Input: part model. Units: mm. Frame: model coordinates. Face numbers are marked on the shaded views. A direction names the side the tool comes from. Coordinates: 2 decimals unless noted, no trailing zeros. Loops run counter-clockwise (first coordinate to the right, second up) from the corner with the lowest first, then second, coordinate; pieces in that order, holes last. Notation, with made-up numbers: (40, -20) -> (55, -20) arc R25 cw to (55, 14) -> close; hole circle Ø5 at (37, 26). An arc over 180 degrees is marked (long way). Put each result on its own line as item: value. Start each with the question number.
1) Set-up query: the marked faces 1 and 2. Return all of +Z, -Z, +X, -X, +Y, -Y with unobstructed straight access to the full face (end or side cutting, diameter ignored); none if empty.
2) Contact query for flat-ended pins moving along their axis: P1, Ø3, axis at y = -1.5, z = 3, coming from the +X side; P2, Ø1, axis at y = -0.5, z = 2.5, coming from the -X side. Output: stop coordinate, or through.
3) Cut plane C-C (z = 4.75). Return the cut outline in (x, y), plus the area to 3 significant figures.
4) Material intervals for L1, parallel to Z at x = -1.65, y = -0.6; L2, parallel to Y at x = 0, z = 4.5; L3, parallel to Y at x = 0.85, z = 4.75, sorted ascending.
5) Cut plane A-A (x = 0). Return the cut outline in (y, z).
from build123d import *

# Parameters (mm, degrees)
SKETCH1_R           = 1.5
BOSS_EXTRUDE1_DEPTH = 6.5
CHAMFER1_SIZE       = 0.1
SKETCH2_R           = 2.5
BOSS_EXTRUDE2_DEPTH = 1
CHAMFER2_SIZE       = 0.2


with BuildPart() as part:
    # Sketch1 → Boss-Extrude1 (new body)
    with BuildSketch(Plane.XY):
        Circle(SKETCH1_R)
    extrude(amount=BOSS_EXTRUDE1_DEPTH)

    # Chamfer1
    chamfer1_edges = [part.edges().sort_by_distance(p)[0] for p in [
        (-1.5, 0, 0),
    ]]
    chamfer(chamfer1_edges, length=CHAMFER1_SIZE)

    # Sketch2 → Boss-Extrude2 (add)
    with BuildSketch(Plane.XY.offset(6.5)):
        Circle(SKETCH2_R)
    extrude(amount=BOSS_EXTRUDE2_DEPTH)

    # Chamfer2
    chamfer2_edges = [part.edges().sort_by_distance(p)[0] for p in [
        (-2.5, 0, 7.5),
    ]]
    chamfer(chamfer2_edges, length=CHAMFER2_SIZE)


solid = part.part
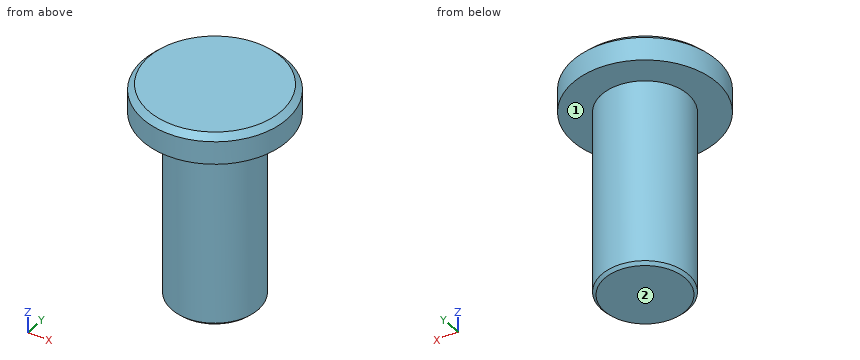
Results found:
1. face 1: -Z
1. face 2: -Z, +X, -X, +Y, -Y
2. P1: stops at x = 1.5
2. P2: stops at x = -1.5
3. outline: circle Ø3 at (0, 0)
3. area: 7.07 mm2
4. L1: z = 6.5 to 7.5
4. L2: y = -1.5 to 1.5
4. L3: y = -1.24 to 1.24
5. outline: (-2.5, 6.5) -> (-1.5, 6.5) -> (-1.5, 0.1) -> (-1.4, 0) -> (1.4, 0) -> (1.5, 0.1) -> (1.5, 6.5) -> (2.5, 6.5) -> (2.5, 7.3) -> (2.3, 7.5) -> (-2.3, 7.5) -> (-2.5, 7.3) -> close
